```python
from build123d import *

# Parameters (mm, degrees)
SKETCH_1_W           = 113
SKETCH_1_H           = 52.5
SKETCH_1_R           = 23.75
EXTRUDE_1_DEPTH      = 2
SKETCH_2_W           = 113
SKETCH_2_H           = 2
EXTRUDE_2_DEPTH      = 11
FILLET_1_R           = 2
SKETCH_3_W           = 4
SKETCH_3_H           = 52.5
EXTRUDE_3_DEPTH      = 20
EXTRUDE_4_DEPTH      = 11
SKETCH_5_W           = 4
SKETCH_5_H           = 22
EXTRUDE_5_DEPTH      = 15
EXTRUDE_5_DEPTH_BACK = 67.5
FILLET_2_R           = 2


with BuildPart() as part:
    # 스케치1 → 보스-돌출1 (new body)
    with BuildSketch(Plane.XY):
        with Locations((56.5, 26.25)):
            Rectangle(SKETCH_1_W, SKETCH_1_H)
        with Locations((88, 25)):
            Circle(SKETCH_1_R, mode=Mode.SUBTRACT)
        with Locations((37.5, 25)):
            Circle(SKETCH_1_R, mode=Mode.SUBTRACT)
    extrude(amount=EXTRUDE_1_DEPTH)

    # 스케치2 → 보스-돌출2 (add)
    with BuildSketch(Plane(origin=(0, 0, 0), x_dir=(-1, 0, 0), z_dir=(0, 0, -1))):
        with Locations((-56.5, 51.5)):
            Rectangle(SKETCH_2_W, SKETCH_2_H)
    extrude(amount=EXTRUDE_2_DEPTH)

    # 필렛1
    fillet_1_edges = [part.edges().sort_by_distance(p)[0] for p in [
        (113, 0, 1),
        (113, 52.5, -4.5),
    ]]
    fillet(fillet_1_edges, radius=FILLET_1_R)

    # 스케치3 → 보스-돌출3 (add)
    with BuildSketch(Plane(origin=(0, 0, 0), x_dir=(-1, 0, 0), z_dir=(0, 0, -1))):
        with Locations((-2, 26.25)):
            Rectangle(SKETCH_3_W, SKETCH_3_H)
    extrude(amount=EXTRUDE_3_DEPTH)

    # 스케치4 → 보스-돌출4 (add)
    with BuildSketch(Plane(origin=(0, 0, 0), x_dir=(-1, 0, 0), z_dir=(0, 0, -1))):
        Polygon((-4, 0), (-4, 50.5), (-12, 50.5), (-12, 25), (-12, 0), align=None)
    extrude(amount=EXTRUDE_4_DEPTH)

    # 스케치5 → 보스-돌출5 (add, two sides)
    with BuildSketch(Plane(origin=(0, 52.5, 0), x_dir=(1, 0, 0), z_dir=(0, 1, 0))) as extrude_5_sk:
        with Locations((2, 9)):
            Rectangle(SKETCH_5_W, SKETCH_5_H)
    extrude(amount=EXTRUDE_5_DEPTH)
    extrude(extrude_5_sk.sketch, amount=-EXTRUDE_5_DEPTH_BACK)

    # 필렛2
    fillet_2_edges = [part.edges().sort_by_distance(p)[0] for p in [
        (4, -15, -9),
        (4, 67.5, -9),
    ]]
    fillet(fillet_2_edges, radius=FILLET_2_R)


solid = part.part
```
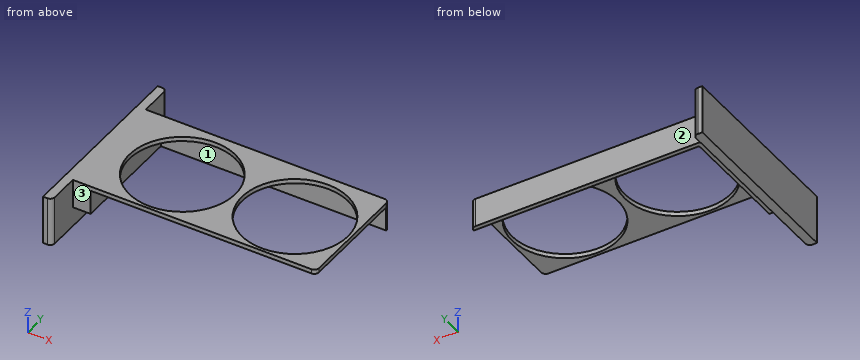
The listing builds one solid part. Answer for the finished solid, in the listing's coordinates (mm). Face numbers are marked on the shaded views. A direction names the side the tool comes from. Round coordinates to 2 decimals unless told otherwise and drop trailing zeros. Write each loop counter-clockwise with the first axis right and the second up, starting at its lowest first coordinate (ties: lowest second). Pieces come first, ordered by that corner, then holes. Notation, with made-up numbers: (47.25, 61) -> (90.25, 61) arc R23 cw to (90.25, 72) -> close; hole circle Ø10 at (55, -32.75). An arc over 180 degrees is marked (long way). Write item = value, one per line.
1) Straight lines are drawn through the part: line 1 along Y through (x, z) = (37.5, 1.4); line 2 along Z through (x, y) = (66.5, 11.5); line 3 along X through (y, z) = (59.5, -10.5). For each, find the intervals that lie inside material, in ascending order. Write a range as [from, to].
Check values:
line_1 = [0, 1.25], [48.75, 52.5]
line_2 = [0, 2]
line_3 = [0, 4]
2) Section D-D on x = 88 is taken. Write down the section's boundary in (y, z).
Check values:
outline = (0, 0) -> (1.25, 0) -> (1.25, 2) -> (0, 2) -> close; (48.75, 0) -> (50.5, 0) -> (50.5, -11) -> (52.5, -11) -> (52.5, 2) -> (48.75, 2) -> close
3) Section B-B on y = 25 is taken. Write down the section's boundary in (x, z).
Check values:
outline = (0, -20) -> (4, -20) -> (4, -11) -> (12, -11) -> (12, 0) -> (13.75, 0) -> (13.75, 2) -> (0, 2) -> close; (61.25, 0) -> (64.25, 0) -> (64.25, 2) -> (61.25, 2) -> close; (111.75, 0) -> (113, 0) -> (113, 2) -> (111.75, 2) -> close
4) Which of the six approach directions +Z, -Z, +X, -X, +Y, -Y give full straight-line access (tool end or side, diameter ignored) to the marked faces 1, 2 and 3?
Check values:
face_1 = -Z, +X, -Y
face_2 = +Z, -Z, +X, +Y
face_3 = +Z, -Z, +X, -Y
5) Given pin 1 (2 mm diameter, centred on y = 39.5, z = -7, fed in from +X); pin 2 (2 mm diameter, centred on x = 60, z = -13, fed in from -Y); pin 3 (4 mm diameter, centred on x = 29, z = -6.5, fed in from +Y); pin 4 (9 mm diameter, centred on x = 55.5, z = -3.5, fed in from -Y), each flat-ended and moving along its own axis, determine where each tip first touches the part or whether it passes through.
Check values:
pin_1 = 12
pin_2 = through
pin_3 = 52.5
pin_4 = 0
6) Section C-C on z = -5.75 is taken. Write down the section's boundary in (x, y), plus the area to 3 significant figures.
Check values:
outline = (0, -15) -> (2, -15) arc R2 ccw to (4, -13) -> (4, 0) -> (12, 0) -> (12, 50.5) -> (113, 50.5) arc R2 ccw to (111, 52.5) -> (4, 52.5) -> (4, 65.5) arc R2 ccw to (2, 67.5) -> (0, 67.5) -> close
area = 949 mm²
7) Section A-A on x = 69 is taken. Write down the section's boundary in (y, z), plus the area to 3 significant figures.
Check values:
outline = (0, 0) -> (10.75, 0) -> (10.75, 2) -> (0, 2) -> close; (39.25, 0) -> (50.5, 0) -> (50.5, -11) -> (52.5, -11) -> (52.5, 2) -> (39.25, 2) -> close
area = 70.0 mm²
